from build123d import *

# Parameters (mm, degrees)
F1_DEPTH = 25.4
F2_W     = 25.4
F2_H     = 25.4
F3_DEPTH = 127
F4_W     = 25.4
F4_H     = 25.4
F5_DEPTH = 114.3


with BuildPart() as f1:
    # F0 (on Front) → F1 (new body)
    with BuildSketch(Plane.XZ):
        Polygon((107.95, -584.2), (107.95, 609.6), (82.55, 609.6), (82.55, -584.2), (-82.55, -584.2), (-82.55, 609.6), (-107.95, 609.6), (-107.95, -584.2), (-107.95, -609.6), (-82.55, -609.6), (82.55, -609.6), (107.95, -609.6), align=None)
    extrude(amount=F1_DEPTH)

    # F2 (on face) → F3 (join)
    with BuildSketch(Plane.XZ.offset(25.4)):
        with Locations((-69.85, -596.9)):
            Rectangle(F2_W, F2_H)
        with Locations((69.85, -596.9)):
            Rectangle(F2_W, F2_H)
    extrude(amount=F3_DEPTH)

    # F4 (on face) → F5 (join)
    with BuildSketch(Plane.YZ.offset(-57.15)):
        with Locations((-63.5, -596.9)):
            Rectangle(F4_W, F4_H)
    extrude(amount=F5_DEPTH)


solid = f1.part
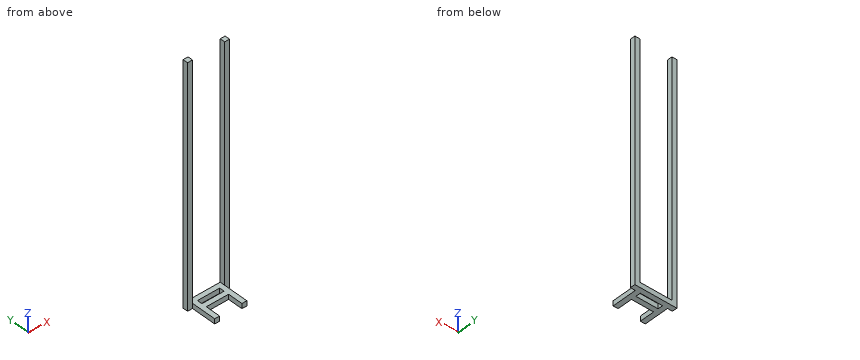
Verification items for the finished model (mm, model axes). Give positions to 0.01 mm unless a question says otherwise; leave off trailing zeros. Loops run counter-clockwise (first coordinate to the right, second up) from the corner with the lowest first, then second, coordinate; pieces in that order, holes last.
1) Thickness scan on line 1 along Z through (x, y) = (-70.5, -42); line 2 along Y through (x, z) = (-92.5, 71); line 3 along X through (y, z) = (-20, -445.5). Record the ranges inside material, lowest first.
2) Sectioned sample at B-B, the plane y = -131. Enter the section's corners in (x, z).
3) Depth check by flat-ended pin: pin 1 Ø12.5 at (x, z) = (-92, 252.5) entering from -Y; pin 2 Ø7.5 at (y, z) = (-108.5, -600) entering from +X; pin 3 Ø7.5 at (y, z) = (-82.5, -596.5) entering from -X. Enter the tip coordinate at first touch or a pass-through.
4) Sectioned sample at A-A, the plane z = -474.5. Enter the section's corners in (x, y).
5) Sectioned sample at C-C, the plane y = -63. Enter the section's corners in (x, z), then the cut area to 3 significant figures.
Answers:
1. line 1: z = -609.6 to -584.2
1. line 2: y = -25.4 to 0
1. line 3: x = -107.95 to -82.55, 82.55 to 107.95
2. outline: (-82.55, -609.6) - (-57.15, -609.6) - (-57.15, -584.2) - (-82.55, -584.2) - close; (57.15, -609.6) - (82.55, -609.6) - (82.55, -584.2) - (57.15, -584.2) - close
3. pin 1: stops at y = -25.4
3. pin 2: stops at x = 82.55
3. pin 3: stops at x = -82.55
4. outline: (-107.95, -25.4) - (-82.55, -25.4) - (-82.55, 0) - (-107.95, 0) - close; (82.55, -25.4) - (107.95, -25.4) - (107.95, 0) - (82.55, 0) - close
5. outline: (-82.55, -609.6) - (82.55, -609.6) - (82.55, -584.2) - (-82.55, -584.2) - close
5. area: 4,190 mm2
